```python
from build123d import *

# Parameters (mm, degrees)
SSS_W               = 37
SSS_H               = 40
SSS_R               = 2.1
BOSS_EXTRUDE2_DEPTH = 3
SKETCH1_W           = 40
SKETCH1_H           = 37
SKETCH1_R           = 2.125
BOSS_EXTRUDE3_DEPTH = 4
BOSS_EXTRUDE4_DEPTH = 4
FILLET1_R           = 2


with BuildPart() as part:
    # sss → Boss-Extrude2 (new body)
    with BuildSketch(Plane(origin=(0, 0, 0), x_dir=(1, 0, 0), z_dir=(0, 1, 0))):
        with Locations((-1.5, 0)):
            Rectangle(SSS_W, SSS_H)
        with Locations(Location((-12, 12, 0), (0, 0, 270))):
            Circle(SSS_R, mode=Mode.SUBTRACT)
        with Locations(Location((12, 12, 0), (0, 0, 90))):
            Circle(SSS_R, mode=Mode.SUBTRACT)
        with Locations(Location((12, -12, 0), (0, 0, 270))):
            Circle(SSS_R, mode=Mode.SUBTRACT)
        with Locations(Location((-12, -12, 0), (0, 0, 90))):
            Circle(SSS_R, mode=Mode.SUBTRACT)
    extrude(amount=BOSS_EXTRUDE2_DEPTH)

    # Sketch1 → Boss-Extrude3 (add)
    with BuildSketch(Plane.ZY.offset(20)):
        with Locations((0, 18.5)):
            Rectangle(SKETCH1_W, SKETCH1_H)
        with Locations((-12, 32)):
            Circle(SKETCH1_R, mode=Mode.SUBTRACT)
        with Locations(Location((12, 32, 0), (0, 0, 180))):
            Circle(SKETCH1_R, mode=Mode.SUBTRACT)
        with Locations((12, 8)):
            Circle(SKETCH1_R, mode=Mode.SUBTRACT)
        with Locations(Location((-12, 8, 0), (0, 0, 180))):
            Circle(SKETCH1_R, mode=Mode.SUBTRACT)
    extrude(amount=-BOSS_EXTRUDE3_DEPTH)

    # Sketch2 → Boss-Extrude4 (add)
    with BuildSketch(Plane.XY.offset(20)):
        Polygon((-20, 37), (-20, 0), (17, 0), (17, 3), (-16, 37), align=None)
    boss_extrude4 = extrude(amount=-BOSS_EXTRUDE4_DEPTH)

    # Mirror1: Boss-Extrude4 across plane
    add(boss_extrude4.mirror(Plane.XY))

    # Fillet1
    fillet1_edges = [part.edges().sort_by_distance(p)[0] for p in [
        (0.5, 3, 16),
        (-16, 3, 0),
        (0.5, 3, -16),
    ]]
    fillet(fillet1_edges, radius=FILLET1_R)


solid = part.part
```
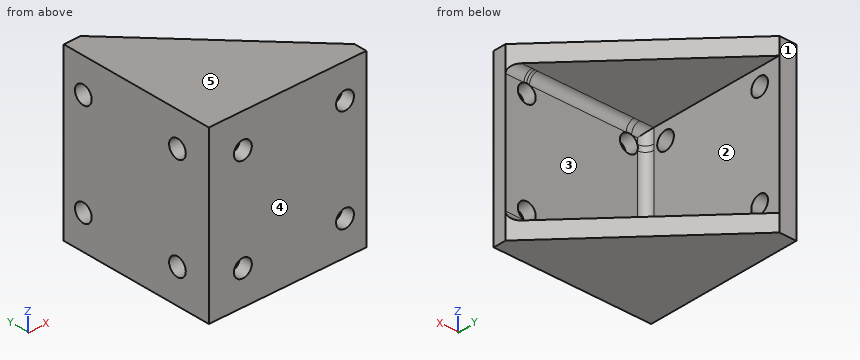
Could you check a few things on this model? Use its own coordinates, in mm. Face numbers are marked on the shaded views. A direction names the side the tool comes from. Round coordinates to 2 decimals unless told otherwise and drop trailing zeros. Loops run counter-clockwise (first coordinate to the right, second up) from the corner with the lowest first, then second, coordinate; pieces in that order, holes last.
Q1. I want a section at B-B (y = 8). Write out the boundary of the cut face in (x, z) (3 decimals), and give its area (3 significant figures).
Q2. For P1, Ø5, axis at x = -3.5, z = 15.5, coming from the +Y side; P2, Ø4, axis at y = 8, z = -12, coming from the -X side; P3, Ø14, axis at x = -2.5, z = 5.5, coming from the +Y side; P4, Ø7, axis at y = 8, z = 12, coming from the +X side, each with a flat end and sliding along its axis, tell me the tip position at first contact or that it passes through.
Q3. I want a section at A-A (z = 7.5). Write out the boundary of the cut face in (x, y).
Q4. I want a section at C-C (x = -17). Write out the boundary of the cut face in (y, z) (3 decimals).
Q5. Thinking about a two-plate mould opening in Z: for the marked faces 3, 4 and 5, which applies, pulls with the +Z half, pulls with the -Z half, needs draft (parallel to the pull), parting line crosses it, or undercut?
Q6. On a 3-axis mill with a long thin cutter (end or side, diameter ignored), from which of +Z, -Z, +X, -X, +Y, -Y can I reach the whole of each face in a straight line? I mean the marked faces 1 and 2. Say none if no direction works.
Q7. I want a section at D-D (z = -12). Give the number of separate pieces and of enclosed holes in the cut face, and give its area (3 significant figures).
Q8. Please list where these lines run through material, in increasing order: L1, parallel to Z at x = 12, y = 1.55; L2, parallel to Y at x = -17.4, z = -12 (3 decimals); L3, parallel to X at y = 1.4, z = -12.
Answer below:
1. outline: (-20, -20) - (12.147, -20) - (12.147, -16) - (-16, -16) - (-16, -14.125) - (-20, -14.125) - close; (-20, -9.875) - (-16, -9.875) - (-16, 9.875) - (-20, 9.875) - close; (-20, 14.125) - (-16, 14.125) - (-16, 16) - (12.147, 16) - (12.147, 20) - (-20, 20) - close
1. area: 351 mm2
2. P1: stops at y = 26.64
2. P2: passes through
2. P3: stops at y = 3
2. P4: stops at x = -15.94
3. outline: (-20, 0) - (17, 0) - (17, 3) - (-14, 3) arc R2 cw to (-16, 5) - (-16, 37) - (-20, 37) - close
4. outline: (0, -20) - (37, -20) - (37, 20) - (0, 20) - close; hole circle Ø4.25 at (8, -12); hole circle Ø4.25 at (8, 12); hole circle Ø4.25 at (32, -12); hole circle Ø4.25 at (32, 12)
5. face 3: undercut
5. face 4: needs draft
5. face 5: pulls with the +Z half
6. face 1: +Z, -Z, +X, -X, +Y
6. face 2: +X, +Y
7. separate pieces: 5
7. enclosed holes: 0
7. area: 189 mm2
8. L1: z = -20 to -14.1, -9.9 to 9.9, 14.1 to 20
8. L2: y = 0 to 5.875, 10.125 to 29.875, 34.125 to 37
8. L3: x = -20 to -14.1, -9.9 to 9.9, 14.1 to 17
